```python
from build123d import *

# Parameters (mm, degrees)
PAD_DEPTH       = 12
SKETCH002_R     = 9
PAD001_DEPTH    = 7.2
SKETCH003_R     = 4.5
POCKET_DEPTH    = 2.5
SKETCH004_R     = 2.7
POCKET001_DEPTH = 12.701
CHAMFER_SIZE    = 1.5
FILLET_R        = 8


with BuildPart() as part:
    # Sketch → Pad (new body, symmetric)
    with BuildSketch(Plane.XY):
        Polygon((-110, 0), (-60, 0), (-45.38, 25.322583), (45.38, 25.322583), (60, 0), (110, 0), (110, 6.4), (70, 7), (70, 8), (64.62, 8), (50, 33.322583), (-50, 33.322583), (-64.62, 8), (-70, 8), (-70, 7), (-110, 6.4), align=None)
    extrude(amount=PAD_DEPTH, both=True)

    # Sketch002 → Pad001 (join)
    with BuildSketch(Plane.XZ.offset(-25.322583)):
        Circle(SKETCH002_R)
    extrude(amount=PAD001_DEPTH)

    # Sketch003 (on Face20 of Pad001) → Pocket (cut)
    with BuildSketch(Plane.XZ.offset(-18.122583)):
        Circle(SKETCH003_R)
    extrude(amount=-POCKET_DEPTH, mode=Mode.SUBTRACT)

    # Sketch004 (on Face22 of Pocket) → Pocket001 (cut, through all)
    with BuildSketch(Plane.XZ.offset(-20.622583)):
        Circle(SKETCH004_R)
    extrude(amount=-POCKET001_DEPTH, mode=Mode.SUBTRACT)

    # Chamfer
    chamfer_edges = [part.edges().sort_by_distance(p)[0] for p in [
        (-9, 25.322583, 0),
    ]]
    chamfer(chamfer_edges, length=CHAMFER_SIZE)

    # Fillet
    fillet_edges = [part.edges().sort_by_distance(p)[0] for p in [
        (-110, 3.2, -12),
        (-110, 3.2, 12),
        (110, 3.2, -12),
        (110, 3.2, 12),
    ]]
    fillet(fillet_edges, radius=FILLET_R)


solid = part.part
```
For this review, take the finished solid that the model builds, in its own axes (mm). A direction names the side the tool comes from. Coordinates: 2 decimals unless noted, no trailing zeros. Write each loop counter-clockwise with the first axis right and the second up, starting at its lowest first coordinate (ties: lowest second). Pieces come first, ordered by that corner, then holes.
(1) Add section A-A on x = 0. Give the boundary of the cut face in (y, z).
(2) Wall thickness on probe 1 along Z at (x, y) = (0, 28.75); probe 2 along X at (y, z) = (20.5, 3.25); probe 3 along Y at (x, z) = (45, -8): over which ranges is each line inside the solid? List them lowest first.
(3) Tool access review of faces 5 (the face through (-1.172, 21.012, 8.923)), 6 (the face through (4, 18.123, -4)), 7 (the face through (67, 8, 0)), 8 (the face through (85, 0, 0)), 9 (the face through (1, 33.323, 3)): name each direction out of +Z, -Z, +X, -X, +Y, -Y from which nothing blocks a thin tool from reaching the whole face with its end or side.
(4) For pin 1 Ø10 at (y, z) = (8.5, -4) entering from +X; pin 2 Ø12 at (x, z) = (43.5, -9) entering from -Y; pin 3 Ø3 at (y, z) = (24, -5.5) entering from +X; pin 4 Ø9 at (x, z) = (0, 2.5) entering from -Y, all flat-tipped, find the tip position at first contact; note any pin that passes through.
(5) Add section D-D on x = -77. Give the boundary of the cut face in (y, z) (3 decimals).
(6) Add section C-C on y = 16. Give the boundary of the cut face in (x, z).
(7) The part is to be moulded in two halves that separate along X. For faces 1 (the face through (-11, 25.323, 0)), 2 (the face through (-52.792, 12.484, 0.168)), 3 (the face through (-107.594, 3.214, -9.719)), 4 (the face through (-85, 0, 0)), say which applies: +X half, -X half, draft (parallel to the pull), parting line (faces both ways), or undercut.
Answer sheet:
1. outline: (18.12, -9) - (23.82, -9) - (25.32, -10.5) - (25.32, -12) - (33.32, -12) - (33.32, -2.7) - (20.62, -2.7) - (20.62, -4.5) - (18.12, -4.5) - close; (18.12, 4.5) - (20.62, 4.5) - (20.62, 2.7) - (33.32, 2.7) - (33.32, 12) - (25.32, 12) - (25.32, 10.5) - (23.82, 9) - (18.12, 9) - close
2. probe 1: z = -12 to -2.7, 2.7 to 12
2. probe 2: x = -57.4 to -48.16, -8.39 to -3.11, 3.11 to 8.39, 48.16 to 57.4
2. probe 3: y = 25.32 to 33.32
3. face 5: -Y
3. face 6: +Z, -Z, -Y
3. face 7: +Z, -Z, +X, +Y
3. face 8: +Z, -Z, +X, -X, -Y
3. face 9: +Z, -Z, +X, -X, +Y
4. pin 1: stops at x = 110
4. pin 2: stops at y = 18.19
4. pin 3: stops at x = 56.25
4. pin 4: stops at y = 18.12
5. outline: (0, -12) - (6.895, -12) - (6.895, 12) - (0, 12) - close
6. outline: (-60, -12) - (-50.76, -12) - (-50.76, 12) - (-60, 12) - close; (50.76, -12) - (60, -12) - (60, 12) - (50.76, 12) - close
7. face 1: undercut
7. face 2: undercut
7. face 3: -X half
7. face 4: draft
